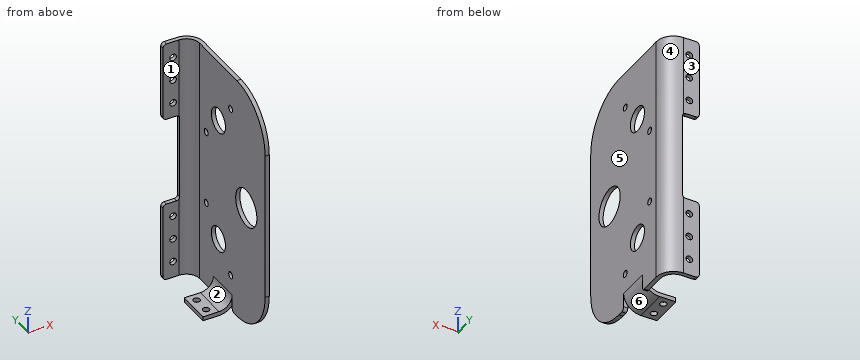
from build123d import *

# Parameters (mm, degrees)
SKETCH1_W                    = 190.5
SKETCH1_H                    = 101.6
BOSS_EXTRUDE1_DEPTH          = 3.175
SKETCH2_R                    = 14.2875
CUT_EXTRUDE1_DEPTH           = 3.175
EDGE_FLANGE1_STRIP_W         = 32.7
EDGE_FLANGE1_STRIP_H         = 3.175
EDGE_FLANGE1_STRIP_CUT_DEPTH = 190.5
EDGE_FLANGE1_DEPTH           = 190.5
SKETCH12_R                   = 9.525
SKETCH12_R_2                 = 2.54
CUT_EXTRUDE2_DEPTH           = 7.62
FILLET1_R                    = 38.1
SKETCH13_W                   = 3.175
SKETCH13_H                   = 25.4
BOSS_EXTRUDE2_DEPTH          = 0.000254
EDGE_FLANGE2_STRIP_W         = 32.7
EDGE_FLANGE2_STRIP_H         = 3.175
EDGE_FLANGE2_STRIP_CUT_DEPTH = 25.4
EDGE_FLANGE2_DEPTH           = 25.4
SKETCH17_R                   = 2.54
CUT_EXTRUDE3_DEPTH           = 142.028796748
SKETCH18_R                   = 2.54
CUT_EXTRUDE4_DEPTH           = 199.405991339
CUT_EXTRUDE5_START           = -34.29
CUT_EXTRUDE5_DEPTH           = 68.58
FILLET3_R                    = 2.54
FILLET4_R                    = 2.54


# Read off the part's stored shape, not the designer's step: Cut-Extrude5
# Sheet-metal steps are written as plain solids
with BuildPart() as part:
    # Sketch1 → Boss-Extrude1 (new body)
    with BuildSketch(Plane(origin=(0, 0, 0), x_dir=(0, 0, -1), z_dir=(1, 0, 0))):
        Rectangle(SKETCH1_W, SKETCH1_H)
    extrude(amount=BOSS_EXTRUDE1_DEPTH)

    # Sketch2 → Cut-Extrude1 (cut)
    with BuildSketch(Plane(origin=(3.175, 0, 0), x_dir=(0, 0, -1), z_dir=(1, 0, 0))):
        with Locations((0, -25.4)):
            Circle(SKETCH2_R)
    extrude(amount=-CUT_EXTRUDE1_DEPTH, mode=Mode.SUBTRACT)

    # Edge-Flange1 strip (across the edge) → Edge-Flange1 strip cut (cut)
    with BuildSketch(Plane(origin=(0, 50.8, 95.25), x_dir=(0, -1, 0), z_dir=(0, 0, -1))):
        with Locations((-3.175, -1.5875)):
            Rectangle(EDGE_FLANGE1_STRIP_W, EDGE_FLANGE1_STRIP_H)
    extrude(amount=EDGE_FLANGE1_STRIP_CUT_DEPTH, mode=Mode.SUBTRACT)

    # Edge-Flange1 section (across the edge) → Edge-Flange1 (add)
    with BuildSketch(Plane(origin=(0, 50.8, 95.25), x_dir=(0, -1, 0), z_dir=(0, 0, -1))):
        with BuildLine():
            Line((0, 10), (0, 22.225))
            Line((0, 22.225), (3.175, 22.225))
            Line((3.175, 22.225), (3.175, 10))
            ThreePointArc((3.175, 10), (6.103932188, 2.928932188), (13.175, 0))
            Line((13.175, 0), (13.175, -3.175))
            ThreePointArc((13.175, -3.175), (3.858868158, 0.683868158), (0, 10))
        make_face()
    extrude(amount=EDGE_FLANGE1_DEPTH)

    # Sketch12 → Cut-Extrude2 (cut)
    with BuildSketch(Plane(origin=(3.175, 0, 0), x_dir=(0, 0, -1), z_dir=(1, 0, 0))):
        with Locations((-47.963329482, 12.225)):
            Circle(SKETCH12_R)
        with Locations((-28.616658964, 28.683017495)):
            Circle(SKETCH12_R_2)
        with Locations((-67.31, -4.233017495)):
            Circle(SKETCH12_R_2)
        with Locations((47.963329482, 12.225)):
            Circle(SKETCH12_R)
        with Locations((28.616658964, 28.683017495)):
            Circle(SKETCH12_R_2)
        with Locations((67.31, -4.233017495)):
            Circle(SKETCH12_R_2)
    extrude(amount=-CUT_EXTRUDE2_DEPTH, mode=Mode.SUBTRACT)

    # Fillet1
    fillet1_edges = [part.edges().sort_by_distance(p)[0] for p in [
        (1.5875, -50.8, 95.25),
        (1.5875, -50.8, -95.25),
    ]]
    fillet(fillet1_edges, radius=FILLET1_R)

    # Sketch13 → Boss-Extrude2 (add)
    with BuildSketch(Plane(origin=(0, 0, -95.25), x_dir=(-1, 0, 0), z_dir=(0, 0, -1))):
        with Locations((-1.5875, 6.35)):
            Rectangle(SKETCH13_W, SKETCH13_H)
    extrude(amount=BOSS_EXTRUDE2_DEPTH)

    # Edge-Flange2 strip (across the edge) → Edge-Flange2 strip cut (cut)
    with BuildSketch(Plane(origin=(0, 19.05, -95.250254), x_dir=(0, 0, 1), z_dir=(0, -1, 0))):
        with Locations((-3.175, -1.5875)):
            Rectangle(EDGE_FLANGE2_STRIP_W, EDGE_FLANGE2_STRIP_H)
    extrude(amount=EDGE_FLANGE2_STRIP_CUT_DEPTH, mode=Mode.SUBTRACT)

    # Edge-Flange2 section (across the edge) → Edge-Flange2 (add)
    with BuildSketch(Plane(origin=(0, 19.05, -95.250254), x_dir=(0, 0, 1), z_dir=(0, -1, 0))):
        with BuildLine():
            Line((0, 10), (0, 22.225))
            Line((0, 22.225), (3.175, 22.225))
            Line((3.175, 22.225), (3.175, 10))
            ThreePointArc((3.175, 10), (6.103932188, 2.928932188), (13.175, 0))
            Line((13.175, 0), (13.175, -3.175))
            ThreePointArc((13.175, -3.175), (3.858868158, 0.683868158), (0, 10))
        make_face()
    extrude(amount=EDGE_FLANGE2_DEPTH)

    # Sketch17 → Cut-Extrude3 (cut, through all)
    with BuildSketch(Plane(origin=(0, 50.8, 0), x_dir=(1, 0, 0), z_dir=(0, 1, 0))):
        with Locations(Location((-14.605, 82.55, 0), (0, 0, 180))):
            Circle(SKETCH17_R)
        with Locations(Location((-14.605, 64.205555556, 0), (0, 0, 180))):
            Circle(SKETCH17_R)
        with Locations(Location((-14.605, 45.861111111, 0), (0, 0, 180))):
            Circle(SKETCH17_R)
        with Locations(Location((-14.605, 27.516666667, 0), (0, 0, 180))):
            Circle(SKETCH17_R)
        with Locations(Location((-14.605, 9.172222222, 0), (0, 0, 180))):
            Circle(SKETCH17_R)
        with Locations(Location((-14.605, -9.172222222, 0), (0, 0, 180))):
            Circle(SKETCH17_R)
        with Locations(Location((-14.605, -27.516666667, 0), (0, 0, 180))):
            Circle(SKETCH17_R)
        with Locations(Location((-14.605, -45.861111111, 0), (0, 0, 180))):
            Circle(SKETCH17_R)
        with Locations(Location((-14.605, -64.205555556, 0), (0, 0, 180))):
            Circle(SKETCH17_R)
        with Locations(Location((-14.605, -82.55, 0), (0, 0, 180))):
            Circle(SKETCH17_R)
    extrude(amount=-CUT_EXTRUDE3_DEPTH, mode=Mode.SUBTRACT)

    # Sketch18 → Cut-Extrude4 (cut, through all)
    with BuildSketch(Plane(origin=(0, 0, -95.250254), x_dir=(-1, 0, 0), z_dir=(0, 0, -1))):
        with Locations((16.35, 12.7)):
            Circle(SKETCH18_R)
        with Locations((16.35, 0)):
            Circle(SKETCH18_R)
    extrude(amount=-CUT_EXTRUDE4_DEPTH, mode=Mode.SUBTRACT)

    # Cut-Extrude5 outline → Cut-Extrude5 (cut)
    with BuildSketch(Plane.XY.offset(CUT_EXTRUDE5_START)):
        with BuildLine():
            ThreePointArc((-10, 47.625), (-9.762432951, 47.622177697), (-9.525, 47.61371238))
            Line((-9.525, 47.61371238), (-9.3741875, 50.78512856))
            ThreePointArc((-9.3741875, 50.78512856), (-9.687005413, 50.796281615), (-10, 50.8))
            Line((-10, 50.8), (-22.225, 50.8))
            Line((-22.225, 50.8), (-22.225, 47.625))
            Line((-22.225, 47.625), (-10, 47.625))
        make_face()
    extrude(amount=CUT_EXTRUDE5_DEPTH, mode=Mode.SUBTRACT)

    # Fillet3
    fillet3_edges = [part.edges().sort_by_distance(p)[0] for p in [
        (-22.225, 49.2125, 95.25),
        (-22.225, 49.2125, 34.29),
        (-9.44959375, 49.19942047, 34.29),
        (-9.44959375, 49.19942047, -34.29),
        (-22.225, 49.2125, -34.29),
        (-22.225, 49.2125, -95.25),
    ]]
    fillet(fillet3_edges, radius=FILLET3_R)

    # Fillet4
    fillet4_edges = [part.edges().sort_by_distance(p)[0] for p in [
        (1.5875, -6.35, -95.25),
        (1.5875, 19.05, -95.25),
    ]]
    fillet(fillet4_edges, radius=FILLET4_R)


solid = part.part
Can you work these out from the model? Positions are in its coordinate system, mm. Face numbers are marked on the shaded views. A direction names the side the tool comes from. Give positions to 0.01 mm unless a question says otherwise; leave off trailing zeros. Loops run counter-clockwise (first coordinate to the right, second up) from the corner with the lowest first, then second, coordinate; pieces in that order, holes last. Notation, with made-up numbers: M 47,-29 L 97,-29 A36 ccw 97,9 Z; hole C 25,15.25 d9. An arc over 180 degrees is marked long. One line per item, written item: value.
1) Imagine slicing it at A-A on x = -6.5. Write out the boundary of the cut face in (y, z).
Geometry check:
outline: M -6.35,-94.78 L 19.05,-94.78 L 19.05,-91.44 L -6.35,-91.44 Z; M 46.99,-95.25 L 50.33,-95.25 L 50.33,95.25 L 46.99,95.25 Z
2) Imagine slicing it at C-C on z = -20. Write out the boundary of the cut face in (x, y) (3 decimals), and give its area (3 significant figures).
Geometry check:
outline: M -9.525,47.614 A10 cw 0,37.625 L 0,-50.8 L 3.175,-50.8 L 3.175,37.625 A13.175 ccw -9.374,50.785 Z
area: 337 mm²
3) On a 3-axis mill with a long thin cutter (end or side, diameter ignored), from which of +Z, -Z, +X, -X, +Y, -Y can I reach the whole of each face in a straight line? I mean the marked faces 1, 2 and 3. Say none if no direction works.
Geometry check:
face 1: +Z, -Z, -X, -Y
face 2: +Z, -X, -Y
face 3: +Z, -Z, +X, -X, +Y
4) Imagine slicing it at B-B on y = -19.5. Write out the boundary of the cut face in (x, z) (3 decimals), and give its area (3 significant figures).
Geometry check:
outline: M 0,-94.638 L 3.175,-94.638 L 3.175,-13.012 L 0,-13.012 Z; M 0,13.012 L 3.175,13.012 L 3.175,94.638 L 0,94.638 Z
area: 518 mm²
5) I'm going to push flat-ended pins straight in: pin 1 (2 mm diameter, centred on x = -7, z = -20.5, fed in from +Y); pin 2 (5 mm diameter, centred on x = -12.5, z = 4.5, fed in from +Y); pin 3 (1 mm diameter, centred on x = 1.5, z = -86, fed in from -Y); pin 4 (1 mm diameter, centred on x = -14.5, y = 5, fed in from +Z). Where does each tip first touch, or does it pass through?
Geometry check:
pin 1: stops at y = 50.65
pin 2: passes through
pin 3: stops at y = -38.15
pin 4: stops at z = -92.08
6) Thinking about a two-plate mould opening in Y: for the marked faces 4, 5 and 6, which applies, +Y half, -Y half, draft (parallel to the pull), parting line (faces both ways), or undercut?
Geometry check:
face 4: +Y half
face 5: draft
face 6: undercut
7) Please list where these lines run through material, in increasing order: line 1 (Y direction, x = -9.5, z = 35); line 2 (X direction, y = 13.5, z = 31) (3 decimals); line 3 (Z direction, x = -13, y = 10.5).
Geometry check:
line 1: y = 47.61 to 50.79
line 2: x = 0 to 3.175
line 3: z = -95.25 to -92.08
